```python
from build123d import *

# Parameters (mm, degrees)
F1_DEPTH  = 58
F3_DEPTH  = 12
F4_R      = 8
F5_DEPTH  = 25
F6_R      = 16
F7_R      = 10
F8_DEPTH  = 12
F9_R      = 15
F9_R_2    = 10
F10_DEPTH = 12
F11_DEPTH = 46
F12_W     = 43
F12_H     = 4
F13_DEPTH = 46
F15_DEPTH = 25


with BuildPart() as f1:
    # F0 (on Top) → F1 (new body)
    with BuildSketch(Plane.XY):
        with BuildLine():
            ThreePointArc((-10, -24), (14.4222051019, -21.6333076528), (26, 0))
            ThreePointArc((26, 0), (14.4222051019, 21.6333076528), (-10, 24))
            Line((-10, 24), (-10, 0))
            Line((-10, 0), (-10, -24))
        make_face()
        with BuildLine():
            ThreePointArc((10, 0), (0, -10), (-10, 0))
            ThreePointArc((-10, 0), (0, 10), (10, 0))
        make_face(mode=Mode.SUBTRACT)
        with BuildLine():
            Line((-10, 0), (-10, 24))
            ThreePointArc((-10, 24), (-26, 0), (-10, -24))
            Line((-10, -24), (-10, 0))
        make_face()
    extrude(amount=F1_DEPTH)

    # F2 (on face) → F3 (join)
    with BuildSketch(Plane(origin=(0, 0, 0), x_dir=(1, 0, 0), z_dir=(0, 0, -1))):
        Polygon((63, 32.5), (0, 32.5), (-63, 32.5), (-63, -32.5), (63, -32.5), align=None)
    extrude(amount=-F3_DEPTH)

    # F4 (on face) → F5 (cut)
    with BuildSketch(Plane.XY.offset(12)):
        with Locations((-50.0454586766, -16.5)):
            Circle(F4_R)
        with Locations((-50.2054683586, 16.5)):
            Circle(F4_R)
        with Locations((45.7945316414, 16.5)):
            Circle(F4_R)
        with Locations((45.9545413234, -16.5)):
            Circle(F4_R)
    extrude(amount=-F5_DEPTH, mode=Mode.SUBTRACT)

    # F6
    f6_edges = [f1.edges().sort_by_distance(p)[0] for p in [
        (-63, 32.5, 6),
        (-63, -32.5, 6),
        (63, 32.5, 6),
        (63, -32.5, 6),
    ]]
    fillet(f6_edges, radius=F6_R)

    # F7 (on face) → F8 (join)
    with BuildSketch(Plane.XY.offset(58)):
        with BuildLine():
            ThreePointArc((26, 0), (8.8317608663, 24.4540385213), (-20, 16.6132477258))
            Line((-20, 16.6132477258), (-20, -16.6132477258))
            ThreePointArc((-20, -16.6132477258), (8.8317608663, -24.4540385213), (26, 0))
        make_face()
        Circle(F7_R, mode=Mode.SUBTRACT)
        with BuildLine():
            ThreePointArc((-20, -22.360679775), (12.2474487139, -27.3861278753), (30, 0))
            ThreePointArc((30, 0), (12.2474487139, 27.3861278753), (-20, 22.360679775))
            Line((-20, 22.360679775), (-20, 16.6132477258))
            ThreePointArc((-20, 16.6132477258), (8.8317608663, 24.4540385213), (26, 0))
            ThreePointArc((26, 0), (8.8317608663, -24.4540385213), (-20, -16.6132477258))
            Line((-20, -16.6132477258), (-20, -22.360679775))
        make_face()
        Circle(F7_R)
        with BuildLine():
            Line((-20, 16.6132477258), (-20, 22.360679775))
            ThreePointArc((-20, 22.360679775), (-30, 0), (-20, -22.360679775))
            Line((-20, -22.360679775), (-20, -16.6132477258))
            ThreePointArc((-20, -16.6132477258), (-26, 0), (-20, 16.6132477258))
        make_face()
        with BuildLine():
            Line((-20, -16.6132477258), (-20, 16.6132477258))
            ThreePointArc((-20, 16.6132477258), (-26, 0), (-20, -16.6132477258))
        make_face()
    extrude(amount=-F8_DEPTH)

    # F9 (on face) → F10 (cut)
    with BuildSketch(Plane.XY.offset(58)):
        Circle(F9_R)
        Circle(F9_R_2, mode=Mode.SUBTRACT)
        Circle(F9_R_2)
    extrude(amount=-F10_DEPTH, mode=Mode.SUBTRACT)

    # F7 (on face) → F11 (cut)
    with BuildSketch(Plane.XY.offset(58)):
        with BuildLine():
            Line((-20, 16.6132477258), (-20, 22.360679775))
            ThreePointArc((-20, 22.360679775), (-30, 0), (-20, -22.360679775))
            Line((-20, -22.360679775), (-20, -16.6132477258))
            ThreePointArc((-20, -16.6132477258), (-26, 0), (-20, 16.6132477258))
        make_face()
        with BuildLine():
            Line((-20, -16.6132477258), (-20, 16.6132477258))
            ThreePointArc((-20, 16.6132477258), (-26, 0), (-20, -16.6132477258))
        make_face()
    extrude(amount=-F11_DEPTH, mode=Mode.SUBTRACT)

    # F12 (on face) → F13 (join)
    with BuildSketch(Plane.XY.offset(12)):
        with Locations((-41.5, 0)):
            Rectangle(F12_W, F12_H)
    extrude(amount=F13_DEPTH)

    # F14 (on face) → F15 (cut)
    with BuildSketch(Plane.XZ.offset(2)):
        Polygon((-63, 12), (-20, 58), (-63, 58), align=None)
    extrude(amount=-F15_DEPTH, mode=Mode.SUBTRACT)


solid = f1.part
```
Part model, mm, in its own coordinate system. A direction names the side the tool comes from. Round coordinates to 2 decimals unless told otherwise and drop trailing zeros. Loops run counter-clockwise (first coordinate to the right, second up) from the corner with the lowest first, then second, coordinate; pieces in that order, holes last. Notation, with made-up numbers: (76.5, 19.5) -> (103.5, 19.5) arc R18 ccw to (103.5, 49.5) -> close; hole circle Ø8 at (-11.75, 0.25). An arc over 180 degrees is marked (long way). Use a Markdown table: item, result.
1) Pull direction X, two halves, no side cores. Call faces 1 (the flat face through (0, 0, 12)), 2 (the flat face through (3, -10, 46)), 3 (the cylindrical face through (-58.437, 27.689, 6.084)), 4 (the flat face through (-32, 2, 24)): pulls with the +X half, pulls with the -X half, needs draft (parallel to the pull), parting line crosses it, or undercut.
The answers:
| item | result |
|---|---|
| face 1 | undercut |
| face 2 | undercut |
| face 3 | pulls with the -X half |
| face 4 | needs draft |
2) Tool access for faces 5 (the flat face through (-20, 10, 35)), 6 (the flat face through (-32, -2, 24)), 7 (the flat face through (27, 0, 12)), 8 (the cylindrical face through (37.962, -16.148, 6.084)): list every direction of +Z, -Z, +X, -X, +Y, -Y with a clear straight run to the whole face (end or side of a thin tool).
The answers:
| item | result |
|---|---|
| face 5 | +Z, -X, +Y |
| face 6 | +Z, -X, -Y |
| face 7 | none |
| face 8 | +Z, -Z |
3) Cut at B-B, the plane x = 0. List the corners of the cut face in (y, z), and give its area (3 significant figures).
The answers:
| item | result |
|---|---|
| outline | (-32.5, 0) -> (32.5, 0) -> (32.5, 12) -> (26, 12) -> (26, 46) -> (30, 46) -> (30, 58) -> (15, 58) -> (15, 46) -> (10, 46) -> (10, 12) -> (-10, 12) -> (-10, 46) -> (-15, 46) -> (-15, 58) -> (-30, 58) -> (-30, 46) -> (-26, 46) -> (-26, 12) -> (-32.5, 12) -> close |
| area | 2,230 mm2 |
4) Probe line 1 (Y direction, x = 0, z = 39); line 2 (Y direction, x = -46.5, z = 5); line 3 (Z direction, x = 11, y = 25). List the from-to ranges inside material, lowest first. Write a range as [from, to].
The answers:
| item | result |
|---|---|
| line 1 | y = [-26, -10], [10, 26] |
| line 2 | y = [-32.5, -23.67], [-9.33, 9.41], [23.59, 32.5] |
| line 3 | z = [0, 12], [46, 58] |
5) Cut at A-A, the plane z = 7. List the corners of the cut face in (x, y).
The answers:
| item | result |
|---|---|
| outline | (-63, -16.5) arc R16 ccw to (-47, -32.5) -> (47, -32.5) arc R16 ccw to (63, -16.5) -> (63, 16.5) arc R16 ccw to (47, 32.5) -> (-47, 32.5) arc R16 ccw to (-63, 16.5) -> close; hole circle Ø16 at (-50.21, 16.5); hole circle Ø16 at (-50.05, -16.5); hole circle Ø16 at (45.79, 16.5); hole circle Ø16 at (45.95, -16.5) |
6) Drop flat-ended pins along their axis: pin 1 Ø23 at (x, y) = (0, 0) entering from +Z; pin 2 Ø10 at (y, z) = (8, 34) entering from -X; pin 3 Ø2 at (x, z) = (-46, 34) entering from -Y; pin 4 Ø8 at (y, z) = (5.5, 23.5) entering from -X. Give the stop position or say it passes through.
The answers:
| item | result |
|---|---|
| pin 1 | stops at z = 46 |
| pin 2 | stops at x = -20 |
| pin 3 | passes through |
| pin 4 | stops at x = -54.06 |
7) Cut at C-C, the plane z = 25.5. List the corners of the cut face in (x, y), and give its area (3 significant figures).
The answers:
| item | result |
|---|---|
| outline | (-50.38, -2) -> (-20, -2) -> (-20, -16.61) arc R26 ccw (long way) to (-20, 16.61) -> (-20, 2) -> (-50.38, 2) -> close; hole circle Ø20 at (0, 0) |
| area | 1,790 mm2 |
8) Cut at D-D, the plane x = -48.5. List the corners of the cut face in (y, z), and give its area (3 significant figures).
The answers:
| item | result |
|---|---|
| outline | (-32.43, 0) -> (-24.35, 0) -> (-24.35, 12) -> (-32.43, 12) -> close; (-8.65, 0) -> (8.68, 0) -> (8.68, 12) -> (2, 12) -> (2, 27.51) -> (-2, 27.51) -> (-2, 12) -> (-8.65, 12) -> close; (24.32, 0) -> (32.43, 0) -> (32.43, 12) -> (24.32, 12) -> close |
| area | 464 mm2 |
